```python
from build123d import *

# Parameters (mm, degrees)
ESQUISSE1_R                     = 2.5
BOSS_EXTRU_1_DEPTH              = 2.5
TROU_TARAUD_M3X0_51_D           = 2.5
TROU_TARAUD_M3X0_51_DEPTH       = 12.5
TROU_TARAUD_M3X0_51_CSINK_D     = 3.05
TROU_TARAUD_M3X0_51_CSINK_ANGLE = 90
TROU_TARAUD_M3X0_51_TIP         = 0.751075774


with BuildPart() as part:
    # Esquisse1 → Boss.-Extru.1 (new body, symmetric)
    with BuildSketch(Plane(origin=(0, 0, 0), x_dir=(1, 0, 0), z_dir=(0, 1, 0))):
        with BuildLine():
            Line((-55.6, -5), (0, -5))
            ThreePointArc((0, -5), (5, 0), (0, 5))
            Line((0, 5), (-55.6, 5))
            Line((-55.6, 5), (-55.6, -5))
        make_face()
        Circle(ESQUISSE1_R, mode=Mode.SUBTRACT)
    extrude(amount=BOSS_EXTRU_1_DEPTH, both=True)

    # Trou taraudé M3x0.51
    with Locations(Plane.ZY.offset(55.6)):
        with Locations((0, -0.25)):
            CounterSinkHole(TROU_TARAUD_M3X0_51_D / 2, TROU_TARAUD_M3X0_51_CSINK_D / 2, depth=TROU_TARAUD_M3X0_51_DEPTH, counter_sink_angle=TROU_TARAUD_M3X0_51_CSINK_ANGLE)
            with Locations((0, 0, -(TROU_TARAUD_M3X0_51_DEPTH + TROU_TARAUD_M3X0_51_TIP / 2))):  # 118° drill point
                Cone(0, TROU_TARAUD_M3X0_51_D / 2, TROU_TARAUD_M3X0_51_TIP, mode=Mode.SUBTRACT)


solid = part.part
```
Could you check a few things on this model? Use its own coordinates, in mm. Coordinates: 2 decimals unless noted, no trailing zeros. Loops run counter-clockwise (first coordinate to the right, second up) from the corner with the lowest first, then second, coordinate; pieces in that order, holes last. Notation, with made-up numbers: M 22,64.5 L 51,64.5 A34 cw 51,102.5 Z; hole C -8.5,-4 d5. An arc over 180 degrees is marked long. Put each result on its own line as item: value. Start each with the question number.
(1) Suppose I cut it at A-A on x = -51. Please give me the cut outline in (y, z).
(2) Will this pin go through, and if not, where does the flat tip stop? P1, Ø2, axis at y = -0.25, z = 0, coming from the -X side.
(3) I need wall thicknesses on line 1 (Y direction, x = -49.5, z = 0); line 2 (X direction, y = -0.4, z = -1.75); line 3 (X direction, y = -1.85, z = 0.75). Which ranges of each line are inside material? Lowest first, please. Write a range as from..to.
(4) Thinking about a two-plate mould opening in Y: for faces 1 (the face through (-26, 2.5, 0)), 2 (the face through (-0.54, -0.04, 2.44)), 3 (the face through (-49.13, -1.47, 0.27)), which applies, pulls with the +Y half, pulls with the -Y half, needs draft (parallel to the pull), parting line crosses it, or undercut?
Solutions:
1. outline: M -2.5,-5 L 2.5,-5 L 2.5,5 L -2.5,5 Z; hole C -0.25,0 d2.5
2. P1: stops at x = -42.95
3. line 1: y = -2.5..-1.5, 1..2.5
3. line 2: x = -55.6..-1.79, 1.79..4.68
3. line 3: x = -55.6..-2.38, 2.38..4.94
4. face 1: pulls with the +Y half
4. face 2: needs draft
4. face 3: undercut
